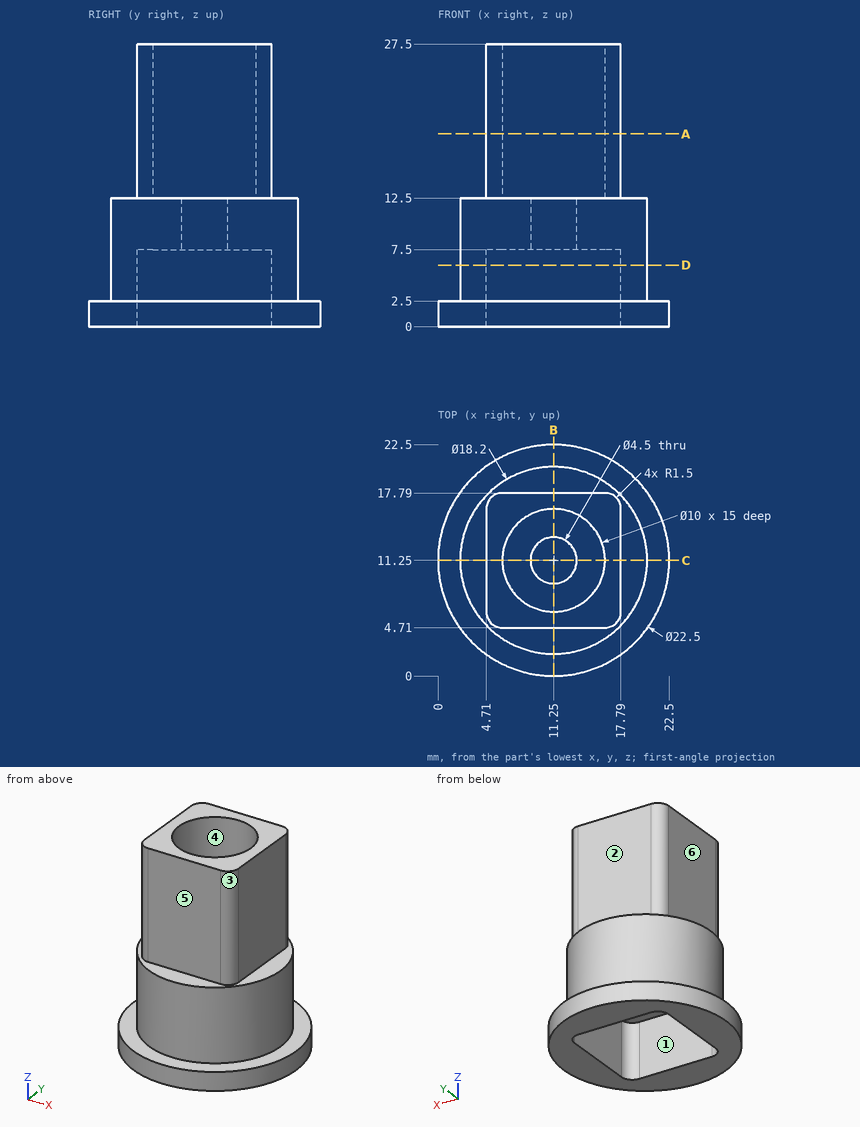
Input: dimensioned drawing with shaded views. Units: mm. Origin: part minimum x, y, z. A direction names the side the tool comes from. Give positions to 0.01 mm unless a question says otherwise; leave off trailing zeros. Write each loop counter-clockwise with the first axis right and the second up, starting at its lowest first coordinate (ties: lowest second). Pieces come first, ordered by that corner, then holes.
1. Section query A-A (z = 18.75). Return the cut outline in (x, y).
2. Section query D-D (z = 6). Return the cut outline in (x, y), then the cut area to 3 significant figures.
3. Section query B-B (x = 11.25). Return the cut outline in (y, z), then the cut area to 3 significant figures.
4. Access query for the marked faces 4, 5 and 6. Directions: +Z, -Z, +X, -X, +Y, -Y. A direction counts if a zero-diameter tool reaches every point of the face in a straight line with its end or side. Return the directions, or none.
5. Pull-direction query (X, two-part tool) for the marked faces 1, 2 and 3; classes: +X half, -X half, draft (parallel to the pull), parting line (faces both ways), or undercut.
6. First-contact query: pin 1 (3 mm diameter, centred on x = 11.5, z = 18, fed in from -Y); pin 2 (12 mm diameter, centred on y = 5, z = 9.5, fed in from -X); pin 3 (2 mm diameter, centred on x = 9, z = 2, fed in from +Y); pin 4 (3.5 mm diameter, centred on x = 11.25, y = 11.25, fed in from -Z). Flat tips, straight axial feed; report the tip coordinate or a pass-through.
7. Material intervals for line 1 along Z through (x, y) = (12, 19.25); line 2 along Y through (x, z) = (11.25, 22); line 3 along Y through (x, z) = (13.5, 26.5), sorted ascending.
Output values:
1. outline: (4.71, 6.21) arc R1.5 ccw to (6.21, 4.71) - (16.29, 4.71) arc R1.5 ccw to (17.79, 6.21) - (17.79, 16.29) arc R1.5 ccw to (16.29, 17.79) - (6.21, 17.79) arc R1.5 ccw to (4.71, 16.29) - close; hole circle Ø10 at (11.25, 11.25)
2. outline: circle Ø18.2 at (11.25, 11.25); hole (4.71, 6.21) arc R1.5 ccw to (6.21, 4.71) - (16.29, 4.71) arc R1.5 ccw to (17.79, 6.21) - (17.79, 16.29) arc R1.5 ccw to (16.29, 17.79) - (6.21, 17.79) arc R1.5 ccw to (4.71, 16.29) - close
2. area: 91.0 mm2
3. outline: (0, 0) - (4.71, 0) - (4.71, 7.5) - (9, 7.5) - (9, 12.5) - (6.25, 12.5) - (6.25, 27.5) - (4.71, 27.5) - (4.71, 12.5) - (2.15, 12.5) - (2.15, 2.5) - (0, 2.5) - close; (13.5, 7.5) - (17.79, 7.5) - (17.79, 0) - (22.5, 0) - (22.5, 2.5) - (20.35, 2.5) - (20.35, 12.5) - (17.79, 12.5) - (17.79, 27.5) - (16.25, 27.5) - (16.25, 12.5) - (13.5, 12.5) - close
3. area: 164 mm2
4. face 4: +Z
4. face 5: +Z, +X, -X, -Y
4. face 6: +Z, -X, +Y, -Y
5. face 1: undercut
5. face 2: draft
5. face 3: +X half
6. pin 1: stops at y = 4.71
6. pin 2: stops at x = 2.15
6. pin 3: stops at y = 22.43
6. pin 4: passes through
7. line 1: z = 0 to 12.5
7. line 2: y = 4.71 to 6.25, 16.25 to 17.79
7. line 3: y = 4.71 to 6.78, 15.72 to 17.79
